```python
from build123d import *

# Parameters (mm, degrees)
BOSS_EXTRUDE1_DEPTH     = 93.8
SKETCH2_W               = 117.3
SKETCH2_H               = 119.6
SKETCH2_R               = 1.5
BOSS_EXTRUDE2_DEPTH     = 2
SKETCH5_W               = 70
SKETCH5_H               = 10
BOSS_EXTRUDE3_DEPTH     = 5
BOSS_EXTRUDE4_DEPTH     = 5
CHAMFER1_SIZE           = 20
BOSS_EXTRUDE5_DEPTH     = 3
CHAMFER2_SIZE2          = 18.660254038
CHAMFER2_SIZE           = 5
FILLET1_R               = 10
SKETCH4_W               = 23.144126226
SKETCH4_H               = 12
CUT_EXTRUDE2_DEPTH      = 221.131710573
CUT_EXTRUDE1_DEPTH      = 192.840558798
CUT_EXTRUDE1_DEPTH_BACK = 192.840558798
SKETCH3_R               = 1.5


with BuildPart() as part:
    # Sketch1 → Boss-Extrude1 (new body)
    with BuildSketch(Plane.XY):
        Polygon((-40, -57.8), (75.3, -57.8), (75.3, 57.8), (-40, 57.8), (-40, 59.8), (77.3, 59.8), (77.3, -59.8), (-40, -59.8), align=None)
    extrude(amount=-BOSS_EXTRUDE1_DEPTH)

    # Sketch2 → Boss-Extrude2 (add)
    with BuildSketch(Plane(origin=(0, 0, -93.8), x_dir=(-1, 0, 0), z_dir=(0, 0, -1))):
        with Locations((-18.65, 0)):
            Rectangle(SKETCH2_W, SKETCH2_H)
        with Locations(Location((33.25, -19.166666667, 0), (0, 0, 90))):
            Circle(SKETCH2_R, mode=Mode.SUBTRACT)
        with Locations(Location((33.25, 19.166666667, 0), (0, 0, 90))):
            Circle(SKETCH2_R, mode=Mode.SUBTRACT)
    extrude(amount=BOSS_EXTRUDE2_DEPTH)

    # Sketch5 → Boss-Extrude3 (add)
    with BuildSketch(Plane(origin=(0, 59.8, 0), x_dir=(1, 0, 0), z_dir=(0, 1, 0))):
        with Locations((-75, 5)):
            Rectangle(SKETCH5_W, SKETCH5_H)
    extrude(amount=-BOSS_EXTRUDE3_DEPTH)

    # Sketch6 → Boss-Extrude4 (add)
    with BuildSketch(Plane(origin=(0, 59.8, 0), x_dir=(1, 0, 0), z_dir=(0, 1, 0))):
        Polygon((-110, 10), (-40, 10), (-40, 30), (77.3, 30), (77.3, 0), (0, 0), (-110, 0), align=None)
    extrude(amount=BOSS_EXTRUDE4_DEPTH)

    # Chamfer1
    chamfer1_edges = [part.edges().sort_by_distance(p)[0] for p in [
        (-40, 61.3, -10),
    ]]
    chamfer(chamfer1_edges, length=CHAMFER1_SIZE)

    # Sketch7 → Boss-Extrude5 (add)
    with BuildSketch(Plane.XZ.offset(-57.8)):
        Polygon((-60, -10), (-40, -30), (-40, -10), align=None)
    extrude(amount=BOSS_EXTRUDE5_DEPTH)

    # Chamfer2
    chamfer2_edges = [part.edges().sort_by_distance(p)[0] for p in [
        (18.65, 59.8, -30),
    ]]
    chamfer2_side = [part.faces().sort_by_distance(p)[0] for p in [
        (18.65, 59.9, -30),
    ]]
    chamfer(chamfer2_edges, length=CHAMFER2_SIZE - 0.0001, length2=CHAMFER2_SIZE2 - 0.0001, reference=chamfer2_side[0])  # a hair under: the kernel refuses the full size

    # Fillet1
    fillet1_edges = [part.edges().sort_by_distance(p)[0] for p in [
        (-110, 59.8, -10),
    ]]
    fillet(fillet1_edges, radius=FILLET1_R - 0.0001)  # a hair under: the kernel refuses the full size

    # Mirror5: part across plane


with BuildPart() as part_1:
    add(part.part)
    add(part.part.mirror(Plane.ZX))

    # Sketch4 → Cut-Extrude2 (cut, through all)
    with BuildSketch(Plane(origin=(77.3, 0, 0), x_dir=(0, 0, -1), z_dir=(1, 0, 0))):
        with Locations((69.25, 36.75)):
            Rectangle(SKETCH4_W, SKETCH4_H)
    extrude(amount=-CUT_EXTRUDE2_DEPTH, mode=Mode.SUBTRACT)

    # Sketch3 → Cut-Extrude1 (cut, two sides: drawn at the far end of the back side and taken through both)
    with BuildSketch(Plane(origin=(0, 59.8, 0), x_dir=(1, 0, 0), z_dir=(0, 1, 0)).offset(-CUT_EXTRUDE1_DEPTH_BACK)):
        with Locations(Location((55, 5, 0), (0, 0, 180))):
            Circle(SKETCH3_R)
        with Locations(Location((-33.25, 5, 0), (0, 0, 180))):
            Circle(SKETCH3_R)
        with Locations(Location((-33.25, 83.5, 0), (0, 0, 270))):
            Circle(SKETCH3_R)
    extrude(amount=CUT_EXTRUDE1_DEPTH + CUT_EXTRUDE1_DEPTH_BACK, mode=Mode.SUBTRACT)


solid = part_1.part
```
Input: part model. Units: mm. Frame: model coordinates. A direction names the side the tool comes from. Round coordinates to 2 decimals unless told otherwise and drop trailing zeros. Loops run counter-clockwise (first coordinate to the right, second up) from the corner with the lowest first, then second, coordinate; pieces in that order, holes last. Notation, with made-up numbers: M 78.25,14 L 98.25,14 A26 ccw 98.25,31 Z; hole C 10,45.5 d7. An arc over 180 degrees is marked long. Answer in a Markdown table with one row per item. Add a question column.
1. Section C-C (y = -32). Output: boundary loops of the cut face in (x, z).
2. Set-up query: faces 4 (the face through (18, 57.8, -46)), 5 (the face through (18, 1, -93.8)), 6 (the face through (-24, 58, 0)), 7 (the face through (-68, -54.8, -8)), 8 (the face through (-80, -60, -10)). Return all of +Z, -Z, +X, -X, +Y, -Y with unobstructed straight access to the full face (end or side cutting, diameter ignored); none if empty.
3. Mould query, pull axis X, two halves, no side actions, for faces 1 (the face through (-50, 60, -20)), 2 (the face through (17, -57.8, -46)), 3 (the face through (19, -59.8, -72)). Classes: released by +X, released by -X, zero draft, split by the parting line, or undercut.
4. Section D-D (z = -45.5). Output: boundary loops of the cut face in (x, y), and give its area (3 significant figures).
5. Ray query, probe 1 along Z at (x, y) = (-33, -58); probe 2 along Y at (x, z) = (39.5, -28.5); probe 3 along X at (y, z) = (61.5, -5). Return the intervals inside material, ascending.
6. Contact query for flat-ended pins moving along their axis: pin 1 (1 mm diameter, centred on x = 42, z = -66, fed in from +Y); pin 2 (8 mm diameter, centred on x = -70.5, y = -57.5, fed in from -Z); pin 3 (1 mm diameter, centred on x = 76.5, y = 39, fed in from +Z); pin 4 (4 mm diameter, centred on x = 51.5, z = -73, fed in from -Y). Output: stop coordinate, or through.
7. Section A-A (z = -16.5). Output: boundary loops of the cut face in (x, y), and give its area (3 significant figures).
Values follow:
| question | item | result |
|---|---|---|
| 1 | outline | M -40,-95.8 L 77.3,-95.8 L 77.3,0 L 75.3,0 L 75.3,-93.8 L -40,-93.8 Z |
| 2 | face 4 | +Z |
| 2 | face 5 | +Z, -X |
| 2 | face 6 | +Z, +X, -X, +Y, -Y |
| 2 | face 7 | +Z, -Z, -X |
| 2 | face 8 | -Z, -X, +Y, -Y |
| 3 | face 1 | released by -X |
| 3 | face 2 | undercut |
| 3 | face 3 | zero draft |
| 4 | outline | M -40,-60.65 L 77.3,-60.65 L 77.3,60.65 L -40,60.65 L -40,57.8 L 75.3,57.8 L 75.3,-57.8 L -40,-57.8 Z |
| 4 | area | 899 mm^2 |
| 5 | probe 1 | -95.8 to -84.98, -82.02 to -6.48, -3.52 to 0 |
| 5 | probe 2 | -64.8 to -57.8, 57.8 to 64.8 |
| 5 | probe 3 | -108.66 to -34.75, -31.75 to 53.5, 56.5 to 77.3 |
| 6 | pin 1 | y = 59.8 |
| 6 | pin 2 | z = -10 |
| 6 | pin 3 | z = 0 |
| 6 | pin 4 | y = -59.8 |
| 7 | outline | M -53.5,-64.8 L 77.3,-64.8 L 77.3,64.8 L -53.5,64.8 L -53.5,54.8 L -40,54.8 L -40,57.8 L 75.3,57.8 L 75.3,-57.8 L -40,-57.8 L -40,-54.8 L -53.5,-54.8 Z |
| 7 | area | 2,140 mm^2 |
